from build123d import *

# Parameters (mm, degrees)
BOSS_EXTRUDE1_DEPTH     = 5
CUT_EXTRUDE2_DEPTH      = 1
CUT_EXTRUDE2_DEPTH_BACK = 1
FILLET1_R               = 1
SKETCH4_R               = 2.15
BOSS_EXTRUDE3_DEPTH     = 10
FILLET2_R               = 1


with BuildPart() as part:
    # Sketch1 → Boss-Extrude1 (new body)
    with BuildSketch(Plane(origin=(0, 0, 0), x_dir=(1, 0, 0), z_dir=(0, 1, 0))):
        with BuildLine():
            Line((-3.9, 3.9), (0, 3.9))
            ThreePointArc((0, 3.9), (2.757716447, 2.757716447), (3.9, 0))
            Line((3.9, 0), (3.9, -3.9))
            Line((3.9, -3.9), (0, -3.9))
            ThreePointArc((0, -3.9), (-2.757716447, -2.757716447), (-3.9, 0))
            Line((-3.9, 0), (-3.9, 3.9))
        make_face()
    extrude(amount=BOSS_EXTRUDE1_DEPTH)

    # Sketch3 → Cut-Extrude2 (cut, two sides: drawn at the far end of the back side and taken through both)
    with BuildSketch(Plane(origin=(0, 2.5, 0), x_dir=(1, 0, 0), z_dir=(0, 1, 0)).offset(-CUT_EXTRUDE2_DEPTH_BACK)):
        with BuildLine():
            Line((-3.9, 0), (-3.9, 3.9))
            Line((-3.9, 3.9), (0, 3.9))
            ThreePointArc((0, 3.9), (2.757716447, 2.757716447), (3.9, 0))
            Line((3.9, 0), (3.9, -3.9))
            Line((3.9, -3.9), (0, -3.9))
            ThreePointArc((0, -3.9), (-2.757716447, -2.757716447), (-3.9, 0))
        make_face()
        with BuildLine():
            Line((-2.9, 0), (-2.9, 2.9))
            Line((-2.9, 2.9), (0, 2.9))
            ThreePointArc((0, 2.9), (2.050609665, 2.050609665), (2.9, 0))
            Line((2.9, 0), (2.9, -2.9))
            Line((2.9, -2.9), (0, -2.9))
            ThreePointArc((0, -2.9), (-2.050609665, -2.050609665), (-2.9, 0))
        make_face(mode=Mode.SUBTRACT)
    extrude(amount=CUT_EXTRUDE2_DEPTH + CUT_EXTRUDE2_DEPTH_BACK, mode=Mode.SUBTRACT)

    # Fillet1
    fillet1_edges = [part.edges().sort_by_distance(p)[0] for p in [
        (2.9, 3.5, 1.45),
        (2.050609665, 3.5, -2.050609665),
        (1.45, 3.5, 2.9),
        (-2.050609665, 3.5, 2.050609665),
        (2.9, 1.5, 1.45),
        (2.050609665, 1.5, -2.050609665),
        (-2.9, 1.5, -1.45),
        (1.45, 1.5, 2.9),
        (-1.45, 3.5, -2.9),
        (-2.9, 3.5, -1.45),
        (-1.45, 1.5, -2.9),
        (-2.050609665, 1.5, 2.050609665),
    ]]
    fillet(fillet1_edges, radius=FILLET1_R - 0.0001)  # a hair under: the kernel refuses the full size

    # Sketch4 → Boss-Extrude3 (add)
    with BuildSketch(Plane(origin=(0, 5, 0), x_dir=(1, 0, 0), z_dir=(0, 1, 0))):
        with BuildLine():
            Line((0, 3.9), (-3.9, 3.9))
            Line((-3.9, 3.9), (-3.9, 0))
            ThreePointArc((-3.9, 0), (-2.757716447, -2.757716447), (0, -3.9))
            Line((0, -3.9), (3.9, -3.9))
            Line((3.9, -3.9), (3.9, 0))
            ThreePointArc((3.9, 0), (2.757716447, 2.757716447), (0, 3.9))
        make_face()
        with Locations(Location((0, 0, 0), (0, 0, 270))):
            Circle(SKETCH4_R, mode=Mode.SUBTRACT)
    extrude(amount=BOSS_EXTRUDE3_DEPTH)

    # Fillet2
    fillet2_edges = [part.edges().sort_by_distance(p)[0] for p in [
        (0, 15, -2.15),
    ]]
    fillet(fillet2_edges, radius=FILLET2_R)


solid = part.part
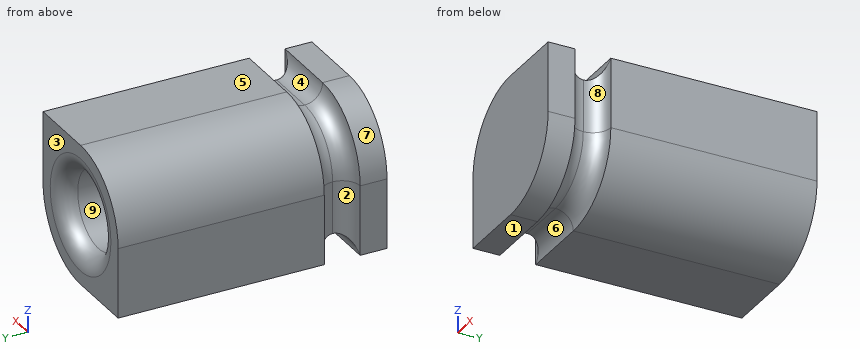
Design review of the part built by this model. Coordinates are the model's own, in mm. Face numbers are marked on the shaded views. A direction names the side the tool comes from. Give positions to 0.01 mm unless a question says otherwise; leave off trailing zeros. One line per question, with ' | ' between items. Start each with the question number.
1. To check wall thickness, follow L1, parallel to Y at x = 1.5, z = -0.5; L2, parallel to X at y = 11.5, z = 1.25; L3, parallel to Y at x = -1.5, z = -3.5. State the ranges of each line that lie inside material, in increasing order.
2. The part is to be moulded in two halves that separate along Y. For the marked faces 1, 2, 3 and 4, say which applies: released by +Y, released by -Y, zero draft, split by the parting line, or undercut.
3. For the marked faces 5, 6, 7, 8 and 9, list the 3-axis set-ups (+Z, -Z, +X, -X, +Y, -Y) from which the entire face can be reached by the end or side of a thin tool; tool diameter is ignored.
4. Insertion check: P1, Ø1, axis at x = 1, y = 5.5, coming from the -Z side; P2, Ø4, axis at x = 0, z = 0, coming from the -Y side; P3, Ø2, axis at y = 6.5, z = 1.5, coming from the -X side; P4, Ø2, axis at x = 0, z = -0.5, coming from the +Y side. Each pin has a flat end and moves straight along its axis. Give the tip position at first contact, or say it passes through.
Worked out:
1) L1: y = 0 to 5 | L2: x = -3.69 to -1.75, 1.75 to 3.9 | L3: y = 0 to 1.58, 3.42 to 15
2) face 1: zero draft | face 2: undercut | face 3: released by +Y | face 4: undercut
3) face 5: +Z, +X, -X, +Y, -Y | face 6: -Z, +X, -X | face 7: +Z, -X, +Y, -Y | face 8: +Z, -Z, +X | face 9: +Y
4) P1: stops at z = -3.87 | P2: stops at y = 0 | P3: stops at x = -3.87 | P4: stops at y = 5
